Verification items for the finished model (mm, model axes). A direction names the side the tool comes from. Coordinates: 2 decimals unless noted, no trailing zeros. Order: outer loops, then holes, each group sorted by start corner. A loop starts at its lowest first (then second) coordinate and runs counter-clockwise, first axis right, second up. Notation, with made-up numbers: M 71.25,27 L 85.25,27 A26 ccw 85.25,55 Z; hole C 21.25,69.25 d5. An arc over 180 degrees is marked long. Answer as a JSON object with one key per item and string values. Group by question number.
(1) Gauge pin test, flat ends, axial feed: pin 1 Ø5 at (x, z) = (5.89, 5) entering from +Y; pin 2 Ø3.5 at (y, z) = (15.5, 5) entering from +X; pin 3 Ø0.5 at (y, z) = (14.5, 5.5) entering from -X. Record the tip position at first contact, or that the pin passes through.
(2) Material ranges on line 1 (Y direction, x = -4.25, z = 3.75); line 2 (Z direction, x = -8.3, y = 27.25) (3 decimals); line 3 (Z direction, x = -9.75, y = 14.65), recorded low to high.
(3) Cross-section at A-A (x = -3.25). Enter the section's corners in (y, z), plus the area to 3 significant figures.
(4) Cross-section at B-B (y = 27.25). Enter the section's corners in (x, z) (3 decimals).
(5) Mould release check, pull along Y, two halves, no side actions. Record for faces 1 (the face through (-6.114, 7, 5)), 2 (the face through (13.393, -2.429, 0.507)), 3 (the face through (-8.63, 31.76, 0.51)): released by +Y, released by -Y, zero draft, split by the parting line, or undercut.
(6) Cross-section at C-C (y = 14.65). Enter the section's corners in (x, z).
(7) Cross-section at D-D (z = 5). Count the separate pieces of the cut face and the enclosed holes in it, plus the area to 3 significant figures.
(8) Access from +Z, -Z, +X, -X, +Y, -Y to the whole of each face (thin tool, end or side, straight path). Record for faces 4 (the face through (-0.114, 16, 5)), 5 (the face through (-1, -5.95, 5)), 6 (the face through (-6.607, 25.827, 9.493)), 7 (the face through (-7.614, 15, 5)), 8 (the face through (-3, 14.25, 5)).
from build123d import *

# Parameters (mm, degrees)
RESSALTO_EXTRUS_O1_DEPTH = 10
ESBO_O3_R                = 2
CORTE_EXTRUS_O1_DEPTH    = 15
CHANFRO1_SIZE            = 1.6
FILETE1_R                = 0.5
CHANFRO5_SIZE            = 2
ESBO_O4_R                = 3.035
CORTE_EXTRUS_O2_DEPTH    = 10
FILETE2_R                = 0.5
CHANFRO6_SIZE            = 1
ESBO_O6_R                = 0.9
CORTE_EXTRUS_O3_DEPTH    = 3.5


with BuildPart() as part:
    # Esboço1 → Ressalto-extrusão1 (new body)
    with BuildSketch(Plane.XY):
        Polygon((-0.113617837, 14.25), (-6.113617837, 14.25), (-6.113617837, -0.95), (13.886382163, -0.95), (13.886382163, -5.95), (-11.113617837, -5.95), (-11.113617837, 32.25), (-6.113617837, 32.25), (-6.113617837, 19.25), (-0.113617837, 19.25), align=None)
    extrude(amount=RESSALTO_EXTRUS_O1_DEPTH)

    # Esboço3 → Corte-extrusão1 (cut)
    with BuildSketch(Plane.XZ.offset(5.95)):
        with Locations(Location((5.886382163, 5, 0), (0, 0, 270))):
            Circle(ESBO_O3_R)
    extrude(amount=-CORTE_EXTRUS_O1_DEPTH, mode=Mode.SUBTRACT)

    # Chanfro1
    chanfro1_edges = [part.edges().sort_by_distance(p)[0] for p in [
        (5.886382163, -5.95, 7),
    ]]
    chamfer(chanfro1_edges, length=CHANFRO1_SIZE)

    # Filete1
    filete1_edges = [part.edges().sort_by_distance(p)[0] for p in [
        (5.886382163, -0.95, 7),
    ]]
    fillet(filete1_edges, radius=FILETE1_R)

    # Chanfro5
    chanfro5_edges = [part.edges().sort_by_distance(p)[0] for p in [
        (13.886382163, -5.95, 5),
        (-11.113617837, -5.95, 5),
        (-0.113617837, 19.25, 5),
    ]]
    chamfer(chanfro5_edges, length=CHANFRO5_SIZE)

    # Esboço4 → Corte-extrusão2 (cut)
    with BuildSketch(Plane(origin=(-6.113617837, 0, 0), x_dir=(0, 0, -1), z_dir=(1, 0, 0))):
        with Locations(Location((-5, 27.25, 0), (0, 0, 90))):
            Circle(ESBO_O4_R)
    extrude(amount=-CORTE_EXTRUS_O2_DEPTH, mode=Mode.SUBTRACT)

    # Filete2
    filete2_edges = [part.edges().sort_by_distance(p)[0] for p in [
        (-11.113617837, 24.215, 5),
        (-6.113617837, 24.215, 5),
    ]]
    fillet(filete2_edges, radius=FILETE2_R)

    # Chanfro6
    chanfro6_edges = [part.edges().sort_by_distance(p)[0] for p in [
        (-11.113617837, 14.15, 0),
        (-8.613617837, 32.25, 0),
        (-6.113617837, 25.75, 10),
        (-6.113617837, 25.75, 0),
        (-0.113617837, 15.75, 0),
        (-8.613617837, 32.25, 10),
        (-11.113617837, 32.25, 5),
        (-6.113617837, 32.25, 5),
        (-6.113617837, 19.25, 5),
        (-11.113617837, 14.15, 10),
        (-4.113617837, 19.25, 0),
        (-4.113617837, 19.25, 10),
        (13.886382163, -2.45, 0),
        (1.386382163, -5.95, 0),
        (12.886382163, -4.95, 0),
        (-10.113617837, -4.95, 0),
        (-1.113617837, 18.25, 0),
        (1.386382163, -5.95, 10),
        (-0.113617837, 15.75, 10),
        (13.886382163, -2.45, 10),
        (12.886382163, -4.95, 10),
        (-10.113617837, -4.95, 10),
        (-1.113617837, 18.25, 10),
    ]]
    chamfer(chanfro6_edges, length=CHANFRO6_SIZE)

    # Esboço6 → Corte-extrusão3 (cut)
    with BuildSketch(Plane.ZY.offset(11.113617837)):
        with Locations(Location((5, 6.65, 0), (0, 0, 270))):
            Circle(ESBO_O6_R)
        with Locations(Location((5, 14.65, 0), (0, 0, 270))):
            Circle(ESBO_O6_R)
    extrude(amount=-CORTE_EXTRUS_O3_DEPTH, mode=Mode.SUBTRACT)


solid = part.part
Taken from the geometry:
{
 "1": {"pin 1": "stops at y = -0.95", "pin 2": "stops at x = -0.11", "pin 3": "stops at x = -7.61"},
 "2": {"line 1": "y = -5.95 to -0.95, 14.25 to 19.25", "line 2": "z = 0 to 1.965, 8.035 to 10", "line 3": "z = 0 to 4.1, 5.9 to 10"},
 "3": {"outline": "M -5.95,1 L -4.95,0 L -0.95,0 L -0.95,10 L -4.95,10 L -5.95,9 Z; M 14.25,0 L 18.25,0 L 19.25,1 L 19.25,9 L 18.25,10 L 14.25,10 Z", "area": "98.0 mm²"},
 "4": {"outline": "M -11.114,1 L -10.114,0 L -7.114,0 L -6.114,1 L -6.114,1.465 A0.5 ccw -6.614,1.965 L -10.614,1.965 A0.5 ccw -11.114,1.465 Z; M -11.114,8.535 A0.5 ccw -10.614,8.035 L -6.614,8.035 A0.5 ccw -6.114,8.535 L -6.114,9 L -7.114,10 L -10.114,10 L -11.114,9 Z"},
 "5": {"face 1": "undercut", "face 2": "zero draft", "face 3": "released by +Y"},
 "6": {"outline": "M -11.11,1 L -10.11,0 L -1.11,0 L -0.11,1 L -0.11,9 L -1.11,10 L -10.11,10 L -11.11,9 L -11.11,5.9 L -7.61,5.9 L -7.61,4.1 L -11.11,4.1 Z"},
 "7": {"separate pieces": "3", "enclosed holes": "0", "area": "249 mm²"},
 "8": {"face 4": "+Z, -Z, +X, +Y", "face 5": "+Z, -Z, +X, -X, -Y", "face 6": "+Z, +X, +Y", "face 7": "-X", "face 8": "+Z, -Z, +X"}
}
